Geometry check sheet. Reference: the model listing, model coordinates, mm. A direction names the side the tool comes from. Coordinates: 2 decimals unless noted, no trailing zeros. Loops run counter-clockwise (first coordinate to the right, second up) from the corner with the lowest first, then second, coordinate; pieces in that order, holes last.
from build123d import *

# Parameters (mm, degrees)
BOSS_EXTRUDE1_DEPTH = 8
SKETCH2_R           = 1.7
CUT_EXTRUDE1_DEPTH  = 19.867962264
FILLET1_R           = 1


with BuildPart() as part:
    # Sketch1 → Boss-Extrude1 (new body)
    with BuildSketch(Plane(origin=(0, 0, 0), x_dir=(1, 0, 0), z_dir=(0, 1, 0))):
        with BuildLine():
            Line((-16, 0), (-8.485281374, 0))
            ThreePointArc((-8.485281374, 0), (-6.753230567, -0.550510257), (-5.656854249, -2))
            ThreePointArc((-5.656854249, -2), (-3.464101615, -4.898979486), (0, -6))
            Line((0, -6), (0, -8))
            ThreePointArc((0, -8), (-4.618802154, -6.531972647), (-7.542472333, -2.666666667))
            ThreePointArc((-7.542472333, -2.666666667), (-7.907931105, -2.183503419), (-8.485281374, -2))
            Line((-8.485281374, -2), (-16, -2))
            Line((-16, -2), (-16, 0))
        make_face()
    extrude(amount=BOSS_EXTRUDE1_DEPTH)

    # Sketch2 → Cut-Extrude1 (cut, through all)
    with BuildSketch(Plane.XY.offset(2)):
        with Locations((-12, 4)):
            Circle(SKETCH2_R)
    extrude(amount=-CUT_EXTRUDE1_DEPTH, mode=Mode.SUBTRACT)

    # Fillet1
    fillet1_edges = [part.edges().sort_by_distance(p)[0] for p in [
        (-16, 4, 0),
        (-16, 4, 2),
    ]]
    fillet(fillet1_edges, radius=FILLET1_R - 0.0001)  # a hair under: the kernel refuses the full size

    # Mirror1: part across plane


with BuildPart() as part_1:
    add(part.part)
    add(part.part.mirror(Plane(origin=(0, 8, 6), x_dir=(0, 0, 1), z_dir=(-1, 0, 0))))


solid = part_1.part
1) Section check B-B on y = 4. Count the separate pieces of the cut face and the enclosed holes in it, and give its area (3 significant figures).
Data:
separate pieces: 3
enclosed holes: 0
area: 59.9 mm2
2) Section check C-C on z = 5. Record the cut outline in (x, y) (3 decimals).
Data:
outline: (-6.245, 0) - (-3.317, 0) - (-3.317, 8) - (-6.245, 8) - close; (3.317, 0) - (6.245, 0) - (6.245, 8) - (3.317, 8) - close
3) Section check D-D on x = -9.5. Record the cut outline in (y, z).
Data:
outline: (0, 0) - (8, 0) - (8, 2) - (0, 2) - close
4) Mould release check, pull along Y, two halves, no side actions. Record for faces 1 (the cylindrical face through (-15.699, 4.056, 0.285)), 2 (the flat face through (-1.3, 0, 6.1)), 3 (the cylindrical face through (-10.43, 3.35, 1.01)): +Y half, -Y half, draft (parallel to the pull), parting line (faces both ways), or undercut.
Data:
face 1: draft
face 2: -Y half
face 3: undercut
5) Section check A-A on x = 12. Record the cut outline in (y, z), and give its area (3 significant figures).
Data:
outline: (0, 0) - (2.3, 0) - (2.3, 2) - (0, 2) - close; (5.7, 0) - (8, 0) - (8, 2) - (5.7, 2) - close
area: 9.20 mm2
6) Depth check by flat-ended pin: pin 1 (1 mm diameter, centred on y = 5.5, z = 5, fed in from -X); pin 2 (3.5 mm diameter, centred on x = 10.5, y = 5, fed in from +Z); pin 3 (3 mm diameter, centred on y = 2.5, z = 2, fed in from -X). Enter the tip coordinate at first touch or a pass-through.
Data:
pin 1: stops at x = -6.61
pin 2: stops at z = 2
pin 3: stops at x = -16
7) Material ranges on probe 1 along Y at (x, z) = (12, 1.05); probe 2 along X at (y, z) = (3.25, 0.5); probe 3 along Z at (x, y) = (12.5, 7.25), recorded low to high.
Data:
probe 1: y = 0 to 2.3, 5.7 to 8
probe 2: x = -15.87 to -13.53, -10.47 to -6.83, 6.83 to 10.47, 13.53 to 15.87
probe 3: z = 0 to 2
8) Access from +Z, -Z, +X, -X, +Y, -Y to the whole of each face (thin tool, end or side, straight path). Record for faces 4 (the cylindrical face through (15.699, 4.056, 0.285)), 5 (the flat face through (10, 4, 2)), 6 (the flat face through (-10, 4, 2)), 7 (the cylindrical face through (6.77, 3.94, 0.54)).
Data:
face 4: -Z, +X, +Y, -Y
face 5: +Z, +X, +Y, -Y
face 6: +Z, -X, +Y, -Y
face 7: -Z, +Y, -Y
